Build history of the part. All positions in model axes, mm. A direction names the side the tool comes from. Give positions to 0.01 mm unless a question says otherwise; leave off trailing zeros. Order: outer loops, then holes, each group sorted by start corner. A loop starts at its lowest first (then second) coordinate and runs counter-clockwise, first axis right, second up. Notation, with made-up numbers: (33.5, 51.25) - (63.5, 51.25) arc R28 ccw to (63.5, 78.25) - close; hole circle Ø6 at (-23, -17.75). An arc over 180 degrees is marked (long way). Use a Markdown table: item, result.
Autodesk Inventor part; units mm, degrees
ref_plane "YZ Plane" through (0, 0, 0) normal (1, 0, 0) x (0, 1, 0)
ref_plane "XZ Plane" through (0, 0, 0) normal (0, 1, 0) x (-1, 0, 0)
ref_plane "XY Plane" through (0, 0, 0) normal (0, 0, 1) x (1, 0, 0)
sketch "Sketch1" plane through (0, 0, 0) normal (0, 0, 1) x (1, 0, 0)
  line L0 (-71, -31) -> (71, -31)
  line L1 (71, -31) -> (71, 31)
  line L2 (71, 31) -> (-71, 31)
  line L3 (-71, 31) -> (-71, -31)
  line L4 (-71, -31) -> (71, 31) construction
  line L5 (71, -31) -> (-71, 31) construction
  line L6 (-73, -33) -> (73, -33)
  line L7 (73, -33) -> (73, 33)
  line L8 (73, 33) -> (-73, 33)
  line L9 (-73, 33) -> (-73, -33)
  line L10 (-73, -33) -> (73, 33) construction
  line L11 (73, -33) -> (-73, 33) construction
  line L12 (-71, 31) -> (71, 31)
  line L13 (71, 31) -> (71, -31)
  line L14 (71, -31) -> (-71, -31)
  line L15 (-71, -31) -> (-71, 31)
  line L16 (-71, 31) -> (71, -31) construction
  line L17 (71, 31) -> (-71, -31) construction
  point P0 (0, 0)
  dimension "d0" = 142
  dimension "d1" = 62
  dimension "d2" = 2
  dimension "d3" = 2
extrude "Extrusion1" add sketch "Sketch1" along normal blind 62
sketch "Sketch2" plane through (0, 0, 0) normal (0, 0, -1) x (-1, 0, 0)
  line L0 (71, -31) -> (-71, -31)
  line L1 (71, 31) -> (-71, 31)
  line L2 (-71, 31) -> (-71, -31)
  line L3 (-71, -31) -> (71, -31)
  line L4 (71, -31) -> (71, 31)
  line L5 (71, 31) -> (-71, -31) construction
  line L6 (-71, 31) -> (71, -31) construction
  point P0 (0, 0)
extrude "Extrusion2" add sketch "Sketch2" against normal blind 2
sketch "Sketch3" plane through (0, 0, 2) normal (0, 0, 1) x (1, 0, 0)
  line L0 (-71, 31) -> (71, 31)
  line L1 (-71, 31) -> (-63, 31)
  line L2 (-63, 31) -> (-63, 23)
  line L3 (-63, 23) -> (-71, 23)
  line L4 (-71, 23) -> (-71, 31)
  line L5 (71, -31) -> (-71, -31)
  line L6 (-71, -31) -> (-63, -31)
  line L7 (-63, -31) -> (-63, -23)
  line L8 (-63, -23) -> (-71, -23)
  line L9 (-71, -23) -> (-71, -31)
  line L10 (71, 31) -> (71, -31)
  line L11 (71, 31) -> (63, 31)
  line L12 (63, 31) -> (63, 23)
  line L13 (63, 23) -> (71, 23)
  line L14 (71, 23) -> (71, 31)
  line L15 (71, 31) -> (71, -31)
  line L16 (71, -31) -> (63, -31)
  line L17 (63, -31) -> (63, -23)
  line L18 (63, -23) -> (71, -23)
  line L19 (71, -23) -> (71, -31)
  point P0 (0, 0)
  dimension "d8" = 8
  dimension "d9" = 8
  dimension "d10" = 8
  dimension "d11" = 8
  dimension "d12" = 8
  dimension "d13" = 8
  dimension "d14" = 8
  dimension "d15" = 8
extrude "Extrusion3" add sketch "Sketch3" along normal blind 55
sketch "Sketch4" plane through (0, 0, 57) normal (0, 0, 1) x (1, 0, 0)
  circle A0 centre (-66, 26) radius 0.9
  circle A1 centre (66, 26) radius 0.9
  circle A2 centre (66, -26) radius 0.9
  circle A3 centre (-66, -26) radius 0.9
  line L0 (-71, 23) -> (-71, 31)
  line L1 (-71, 31) -> (-63, 31)
  line L2 (63, 31) -> (71, 31)
  line L3 (-71, -31) -> (-71, 31)
  point P0 (0, 0)
  dimension "d18" = 1.8
  dimension "d19" = 1.8
  dimension "d20" = 1.8
  dimension "d21" = 1.8
  dimension "d22" = 132
  dimension "d23" = 52
  dimension "d24" = 132
  dimension "d25" = 5
  dimension "d26" = 5
  dimension "d27" = 52
  dimension "d28" = 5
  dimension "d29" = 5
extrude "Extrusion4" cut sketch "Sketch4" against normal blind 20
fillet "Fillet1" radius 2 4 edges at (-73, -33, 31) (73, -33, 31) (73, 33, 31) (-73, 33, 31)
equation "\"d10\" = d8"
equation "\"d11\" = d9"
equation "\"d12\" = d8"
equation "\"d13\" = d9"
equation "\"d14\" = d8"
equation "\"d15\" = d9"
equation "\"d19\" = d18"
equation "\"d20\" = d18"
equation "\"d21\" = d18"
equation "\"d24\" = d22"
equation "\"d25\" = d26"
equation "\"d27\" = d23"
equation "\"d28\" = d26"
equation "\"d29\" = d26"
properties part number "Box"
1) Slice it at B-B (x = -34). Write the cut outline in (y, z), and give its area (3 significant figures).
Computed:
| item | result |
|---|---|
| outline | (-33, 0) - (33, 0) - (33, 62) - (31, 62) - (31, 2) - (-31, 2) - (-31, 62) - (-33, 62) - close |
| area | 372 mm² |
2) Two-plate mould, pull along Y, no slides. Class faces 3 (the flat face through (67, 23, 29)), 4 (the flat face through (0, 32, 62)), 5 (the flat face through (1, 33, 31)): +Y half, -Y half, draft (parallel to the pull), parting line (faces both ways), or undercut.
Computed:
| item | result |
|---|---|
| face 3 | undercut |
| face 4 | draft |
| face 5 | +Y half |
3) Pin check, flat tips, straight feed: P1, Ø2, axis at x = 66, y = -26, coming from the +Z side; P2, Ø3, axis at x = -66, y = -26, coming from the -Z side; P3, Ø1.5, axis at x = 26, y = 19.5, coming from the +Z side. Stop position of each tip, or through.
Computed:
| item | result |
|---|---|
| P1 | stops at z = 57 |
| P2 | stops at z = 0 |
| P3 | stops at z = 2 |
4) Slice it at A-A (z = 47). Write the cut outline in (x, y), and give its area (3 significant figures).
Computed:
| item | result |
|---|---|
| outline | (-73, -31) arc R2 ccw to (-71, -33) - (71, -33) arc R2 ccw to (73, -31) - (73, 31) arc R2 ccw to (71, 33) - (-71, 33) arc R2 ccw to (-73, 31) - close; hole (-71, -23) - (-63, -23) - (-63, -31) - (63, -31) - (63, -23) - (71, -23) - (71, 23) - (63, 23) - (63, 31) - (-63, 31) - (-63, 23) - (-71, 23) - close; hole circle Ø1.8 at (-66, -26); hole circle Ø1.8 at (-66, 26); hole circle Ø1.8 at (66, -26); hole circle Ø1.8 at (66, 26) |
| area | 1,070 mm² |
5) Tool access for faces 1 (the flat face through (-67, -27, 57)), 2 (the flat face through (-1, -33, 31)): list every direction of +Z, -Z, +X, -X, +Y, -Y with a clear straight run to the whole face (end or side of a thin tool).
Computed:
| item | result |
|---|---|
| face 1 | +Z |
| face 2 | +Z, -Z, +X, -X, -Y |
6) Slice it at C-C (z = 14.5). Write the cut outline in (x, y), and give its area (3 significant figures).
Computed:
| item | result |
|---|---|
| outline | (-73, -31) arc R2 ccw to (-71, -33) - (71, -33) arc R2 ccw to (73, -31) - (73, 31) arc R2 ccw to (71, 33) - (-71, 33) arc R2 ccw to (-73, 31) - close; hole (-71, -23) - (-63, -23) - (-63, -31) - (63, -31) - (63, -23) - (71, -23) - (71, 23) - (63, 23) - (63, 31) - (-63, 31) - (-63, 23) - (-71, 23) - close |
| area | 1,080 mm² |
7) Slice it at D-D (y = 13). Write the cut outline in (x, z), and give its area (3 significant figures).
Computed:
| item | result |
|---|---|
| outline | (-73, 0) - (73, 0) - (73, 62) - (71, 62) - (71, 2) - (-71, 2) - (-71, 62) - (-73, 62) - close |
| area | 532 mm² |
8) Wall check: line 1 (Y direction, x = -66, z = 50); line 2 (X direction, y = -29, z = 59); line 3 (X direction, y = 25.5, z = 22). Give the ranges that are in metal, low to high. Write a range as from..to.
Computed:
| item | result |
|---|---|
| line 1 | y = -33..-26.9, -25.1..-23, 23..25.1, 26.9..33 |
| line 2 | x = -73..-71, 71..73 |
| line 3 | x = -73..-63, 63..73 |
